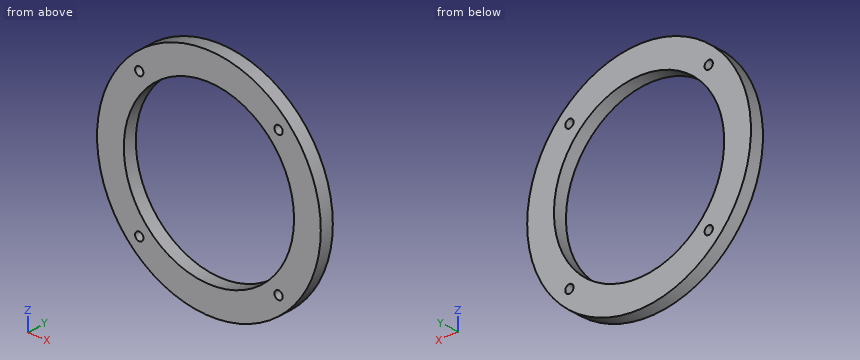
```python
from build123d import *

# Parameters (mm, degrees)
CROQUIS1_R              = 41.8402633
CROQUIS1_R_2            = 1.55
CROQUIS1_R_3            = 31.8402633
SALIENTE_EXTRUIR1_DEPTH = 5


with BuildPart() as part:
    # Croquis1 → Saliente-Extruir1 (new body)
    with BuildSketch(Plane(origin=(0, 0, 0), x_dir=(1, 0, 0), z_dir=(0, 1, 0))):
        Circle(CROQUIS1_R)
        with Locations((-26.05, 26.05)):
            Circle(CROQUIS1_R_2, mode=Mode.SUBTRACT)
        Circle(CROQUIS1_R_3, mode=Mode.SUBTRACT)
        with Locations((26.05, 26.05)):
            Circle(CROQUIS1_R_2, mode=Mode.SUBTRACT)
        with Locations((26.05, -26.05)):
            Circle(CROQUIS1_R_2, mode=Mode.SUBTRACT)
        with Locations((-26.05, -26.05)):
            Circle(CROQUIS1_R_2, mode=Mode.SUBTRACT)
    extrude(amount=SALIENTE_EXTRUIR1_DEPTH)


solid = part.part
```
Part model, mm, in its own coordinate system. Round coordinates to 2 decimals unless told otherwise and drop trailing zeros. Order: outer loops, then holes, each group sorted by start corner. A loop starts at its lowest first (then second) coordinate and runs counter-clockwise, first axis right, second up. Notation, with made-up numbers: M 75.25,72 L 127.25,72 A20 ccw 127.25,79 Z; hole C 4.5,52 d5. An arc over 180 degrees is marked long. Answer in a Markdown table with one row per item. Add a question column.
Q1. Cut at B-B on y = 2.7. Give the cut face in (x, z), and give its area (3 significant figures).
Q2. Cut at A-A on x = 0. Give the cut face in (y, z), and give its area (4 significant figures).
Q3. Wall check: L1, parallel to Z at x = 0, y = 2.35; L2, parallel to X at y = 1.45, z = 26.05. Give the ranges that are in metal, low to high. Write a range as from..to.
Q4. Cut at C-C on z = 0. Give the cut face in (x, y), and give its area (4 significant figures).
Q5. Pin check, flat tips, straight feed: pin 1 (2 mm diameter, centred on x = -17.5, y = 2.5, fed in from -Z); pin 2 (2 mm diameter, centred on x = 2.5, y = 3, fed in from +Z). Stop position of each tip, or through.
Q6. Cut at D-D on x = -26.05. Give the cut face in (y, z).
Established:
| question | item | result |
|---|---|---|
| 1 | outline | C 0,0 d83.68; hole C 0,0 d63.68; hole C -26.05,-26.05 d3.1; hole C -26.05,26.05 d3.1; hole C 26.05,-26.05 d3.1; hole C 26.05,26.05 d3.1 |
| 1 | area | 2,280 mm2 |
| 2 | outline | M 0,-41.84 L 5,-41.84 L 5,-31.84 L 0,-31.84 Z; M 0,31.84 L 5,31.84 L 5,41.84 L 0,41.84 Z |
| 2 | area | 100.0 mm2 |
| 3 | L1 | z = -41.84..-31.84, 31.84..41.84 |
| 3 | L2 | x = -32.74..-27.6, -24.5..-18.31, 18.31..24.5, 27.6..32.74 |
| 4 | outline | M -41.84,0 L -31.84,0 L -31.84,5 L -41.84,5 Z; M 31.84,0 L 41.84,0 L 41.84,5 L 31.84,5 Z |
| 4 | area | 100.0 mm2 |
| 5 | pin 1 | stops at z = -38.45 |
| 5 | pin 2 | stops at z = 41.81 |
| 6 | outline | M 0,-32.74 L 5,-32.74 L 5,-27.6 L 0,-27.6 Z; M 0,-24.5 L 5,-24.5 L 5,-18.31 L 0,-18.31 Z; M 0,18.31 L 5,18.31 L 5,24.5 L 0,24.5 Z; M 0,27.6 L 5,27.6 L 5,32.74 L 0,32.74 Z |
